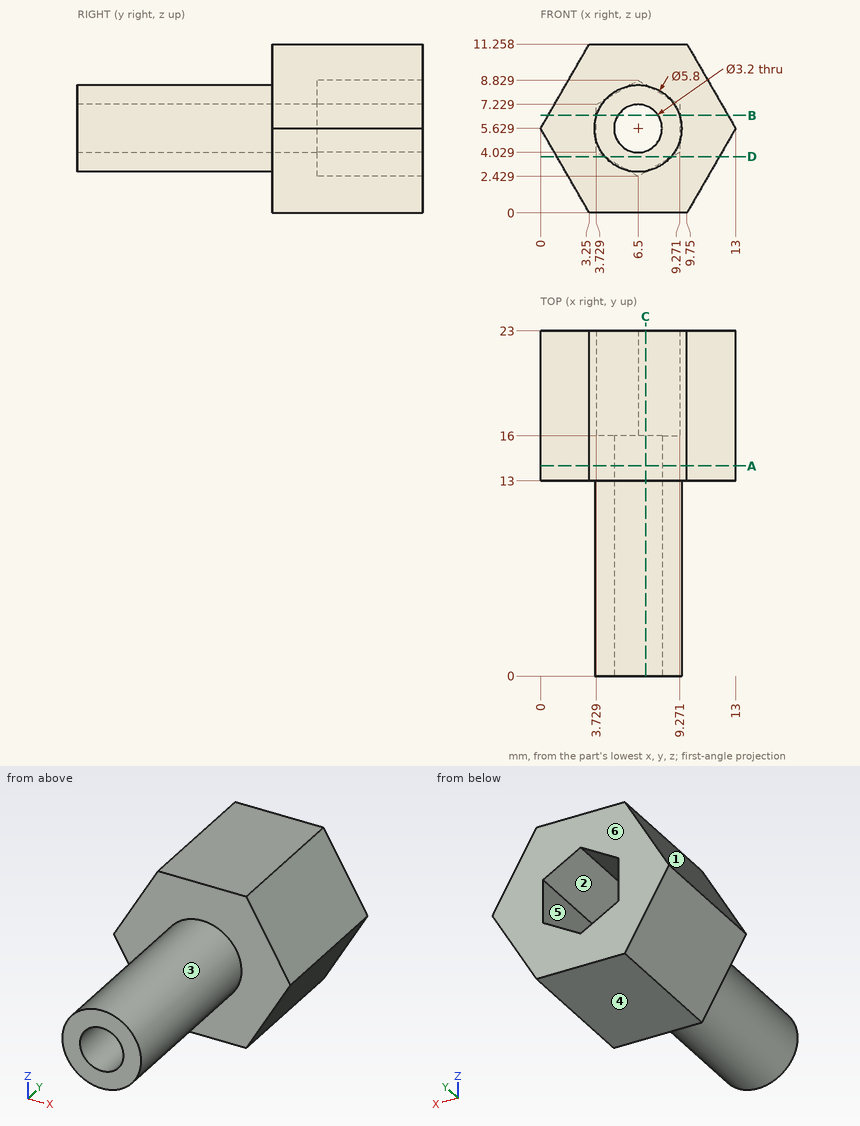
Here's the drawing with two shaded views (mm, measured from the low corner). I have some questions. A direction names the side the tool comes from. Coordinates: 2 decimals unless noted, no trailing zeros. Order: outer loops, then holes, each group sorted by start corner. A loop starts at its lowest first (then second) coordinate and runs counter-clockwise, first axis right, second up.
Item 1: If we section it at C-C, the plane x = 7: List the corners of the cut face in (y, z) for me.
Response values:
outline: (0, 2.77) - (13, 2.77) - (13, 0) - (23, 0) - (23, 2.72) - (16, 2.72) - (16, 4.11) - (0, 4.11) - close; (0, 7.15) - (16, 7.15) - (16, 8.54) - (23, 8.54) - (23, 11.26) - (13, 11.26) - (13, 8.49) - (0, 8.49) - close
Item 2: Which directions (+Z, -Z, +X, -X, +Y, -Y) give clear straight access to the entire face, cutting with the end or side of a thin tool? Please do the marked faces 1, 2 and 3.
Response values:
face 1: +Z, -X, +Y, -Y
face 2: +Y
face 3: -Y
Item 3: Thinking about a two-plate mould opening in Z: for the marked faces 4, 5 and 6, which applies, pulls with the +Z half, pulls with the -Z half, needs draft (parallel to the pull), parting line crosses it, or undercut?
Response values:
face 4: pulls with the -Z half
face 5: undercut
face 6: needs draft
Item 4: If we section it at B-B, the plane z = 6.5: List the corners of the cut face in (x, y) for me, then the cut area to 3 significant figures.
Response values:
outline: (0.5, 13) - (3.73, 13) - (3.73, 0) - (5.16, 0) - (5.16, 16) - (3.73, 16) - (3.73, 23) - (0.5, 23) - close; (7.84, 0) - (9.27, 0) - (9.27, 13) - (12.5, 13) - (12.5, 23) - (9.27, 23) - (9.27, 16) - (7.84, 16) - close
area: 110 mm2
Item 5: I'm going to push flat-ended pins straight in: pin 1 Ø1.5 at (y, z) = (9, 2.5) entering from -X; pin 2 Ø2 at (y, z) = (17, 8) entering from +X; pin 3 Ø3 at (y, z) = (19, 1.5) entering from +X. Where does each tip first touch, or does it pass through?
Response values:
pin 1: stops at x = 4.84
pin 2: stops at x = 12.21
pin 3: stops at x = 11.48
Item 6: If we section it at A-A, the plane y = 14: List the corners of the cut face in (x, z) for me.
Response values:
outline: (0, 5.63) - (3.25, 0) - (9.75, 0) - (13, 5.63) - (9.75, 11.26) - (3.25, 11.26) - close; hole circle Ø3.2 at (6.5, 5.63)
Item 7: If we section it at D-D, the plane z = 3.75: List the corners of the cut face in (x, y) for me (1 decimal).
Response values:
outline: (1.1, 13) - (4.3, 13) - (4.3, 0) - (8.7, 0) - (8.7, 13) - (11.9, 13) - (11.9, 23) - (8.8, 23) - (8.8, 16) - (4.2, 16) - (4.2, 23) - (1.1, 23) - close
Item 8: I need wall thicknesses on probe 1 along X at (y, z) = (7, 5.75) (1 decimal); probe 2 along Y at (x, z) = (12.25, 5.75); probe 3 along Y at (x, z) = (9, 6.25). Which ranges of each line are inside material? Lowest first, please.
Response values:
probe 1: x = 3.6 to 4.9, 8.1 to 9.4
probe 2: y = 13 to 23
probe 3: y = 0 to 16
